Autodesk Inventor part; units mm, degrees
ref_plane "YZ Plane" through (0, 0, 0) normal (1, 0, 0) x (0, 1, 0)
ref_plane "XZ Plane" through (0, 0, 0) normal (0, 1, 0) x (-1, 0, 0)
ref_plane "XY Plane" through (0, 0, 0) normal (0, 0, 1) x (1, 0, 0)
sketch "スケッチ1" plane through (0, 0, 0) normal (0, 0, 1) x (1, 0, 0)
  line L0 (0, 0) -> (0, -3)
  line L1 (0, 0) -> (-15, 0)
  line L2 (-15, 0) -> (-15, -3)
  line L3 (-15, -3) -> (-30, -3)
  line L4 (-30, -3) -> (-30, 0)
  line L5 (-30, 0) -> (-45, 0)
  line L6 (-45, 0) -> (-45, -3)
  line L7 (-245.5996, 0) -> (-66.4062, 0)
  line L8 (-66.4062, 0) -> (-51.9242, -3.906)
  line L9 (-245.5996, 0) -> (-245.5996, -3)
  line L10 (-245.5996, -3) -> (-68.9626, -6)
  line L11 (-68.9626, -6) -> (-58.5737, -15.799)
  circle A0 centre (-53.7535, -10.6886) radius 4.025
  circle A1 centre (-53.7535, -10.6886) radius 1.5
  line L12 (0, -3) -> (0, -9)
  arc A2 (-54.2694, -3.6826) -> (-51.0532, -17.1739) centre (-53.7535, -10.6886) ccw
  line L13 (-54.2694, -3.6826) -> (-45, -3)
  line L14 (-51.0532, -17.1739) -> (-31.4218, -9)
  line L15 (-31.4218, -9) -> (0, -9)
  arc A3 (-46.7293, -10.7926) -> (-42.5418, -13.63) centre (-43.7046, -10.8374) ccw
  circle A4 centre (-43.7046, -10.8374) radius 1.5
  line L16 (-54.6828, -17.6519) -> (-41.7856, -19.3732)
  arc A5 (-41.7856, -19.3732) -> (-42.5418, -13.63) centre (-41.3887, -16.3996) ccw
  arc A6 (-58.5737, -15.799) -> (-54.6828, -17.6519) centre (-53.7535, -10.6886) ccw
  arc A7 (-46.7293, -10.7926) -> (-51.9242, -3.906) centre (-53.7535, -10.6886) ccw
  line L17 (-42, -3) -> (-33, -3)
  line L18 (-33, -3) -> (-33, -6)
  line L19 (-33, -6) -> (-42, -6)
  line L20 (-42, -6) -> (-42, -3)
  line L21 (-12, -3) -> (-3, -3)
  line L22 (-3, -3) -> (-3, -6)
  line L23 (-3, -6) -> (-12, -6)
  line L24 (-12, -6) -> (-12, -3)
  circle A8 centre (-40.95, -3) radius 1.05
  circle A9 centre (-34.05, -3) radius 1.05
  circle A10 centre (-34.05, -6) radius 1.05
  circle A11 centre (-40.95, -6) radius 1.05
  circle A12 centre (-10.95, -3) radius 1.05
  circle A13 centre (-4.05, -3) radius 1.05
  circle A14 centre (-4.05, -6) radius 1.05
  circle A15 centre (-10.95, -6) radius 1.05
  circle A16 centre (-28.95, -3) radius 1.05
  circle A17 centre (-16.05, -3) radius 1.05
  circle A18 centre (-41.3887, -16.3996) radius 1.25
  line L25 (-15.5802, -9) -> (-15.5802, -14)
  line L26 (-15.5802, -14) -> (-4.3492, -14)
  line L27 (-4.3492, -14) -> (-4.3492, -12)
  line L28 (-4.3492, -12) -> (-11.5802, -12)
  arc A19 (-11.5802, -9) -> (-11.5802, -12) centre (-11.5802, -10.5) ccw
  line L29 (-43.7046, -10.8374) -> (-53.7535, -10.6886)
  line L30 (-53.7535, -10.6886) -> (-43.8314, -9.0902)
  arc A20 (-43.0841, -6.159) -> (-46.8179, -9.5713) centre (-43.8314, -9.0902) ccw
  line L31 (-52.0181, -3.8813) -> (-43.0841, -6.159)
  circle A21 centre (-88, 0) radius 0.5
  circle A22 centre (-158, 0) radius 0.5
  circle A23 centre (-228, 0) radius 0.5
  point P0 (-5.1, -6)
  point P1 (-9.9, -6)
  point P2 (-12, -6)
  point P3 (-9.9, -3)
  point P4 (-5.1, -3)
  point P5 (-33, -3)
  point P6 (-33, -6)
  point P7 (-35.1, -6)
  point P8 (-39.9, -6)
  point P9 (-42, -6)
  point P10 (-42, -3)
  point P11 (-39.9, -3)
  point P12 (-35.1, -3)
  point P13 (-17.1, -3)
  point P14 (-27.9, -3)
  point P15 (-58.5737, -15.799)
  point P16 (-54.6828, -17.6519)
  point P17 (-51.9709, -3.8934)
  point P18 (-46.8179, -9.5713)
  point P19 (-87.5, 0)
  point P20 (-88.5, 0)
  point P21 (-157.5, 0)
  point P22 (-158.5, 0)
  point P23 (-227.5, 0)
  point P24 (-228.5, 0)
  dimension "d0" = 3
  dimension "d1" = 15
  dimension "d2" = 3
  dimension "d3" = 15
  dimension "d4" = 15
  dimension "d5" = 3
  dimension "d6" = 3
  dimension "d7" = 8.05
  dimension "d8" = 3
  dimension "d9" = 6
  dimension "d10" = 6
  dimension "d11" = 6.05
  dimension "d12" = 3
  dimension "d13" = 9
  dimension "d14" = 3
  dimension "d15" = 9
  dimension "d16" = 3
  dimension "d17" = 3
  dimension "d18" = 3
  dimension "d19" = 3
  dimension "d20" = 3
  dimension "d21" = 3
  dimension "d22" = 2.1
  dimension "d23" = 2.1
  dimension "d24" = 2.1
  dimension "d25" = 2.1
  dimension "d26" = 2.1
  dimension "d27" = 2.1
  dimension "d28" = 2.1
  dimension "d29" = 2.1
  dimension "d30" = 2.1
  dimension "d31" = 2.1
  dimension "d32" = 2.5
  dimension "d33" = 3
  dimension "d34" = 3
  dimension "d35" = 2
  dimension "d36" = 4
  dimension "d39" = 10
  dimension "d42" = 1
  dimension "d43" = 43
  dimension "d44" = 1
  dimension "d45" = 1
  dimension "d46" = 70
  dimension "d47" = 70
extrude "押し出し1" add sketch "スケッチ1" along normal blind 6 contours A5 L16 A2 L14 | L14 A2 L13 L8 A7 L30 A0 L29 A3 | L29 A0 L30 A7 | A7 L31 A20 | L11 L10 L9 L7 A23 A22 A21 L8 L13 A2
fillet "フィレット1" radius 1 1 edges at (-43.0841, -6.159, 3)
properties part number "シールド先端棒"
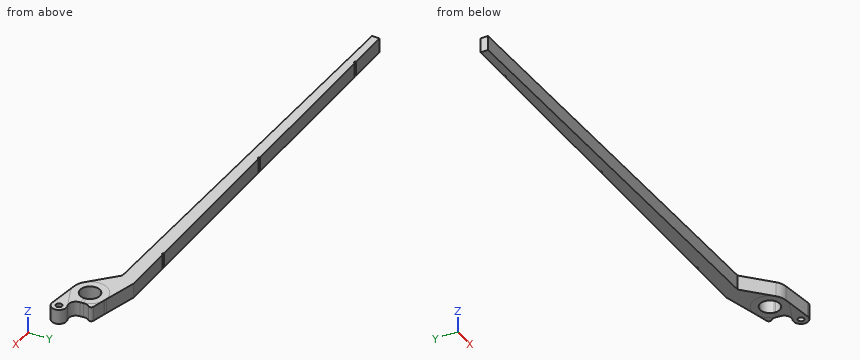
For this review, take the finished solid that the model builds, in its own axes (mm). Round coordinates to 2 decimals unless told otherwise and drop trailing zeros. Order: outer loops, then holes, each group sorted by start corner. A loop starts at its lowest first (then second) coordinate and runs counter-clockwise, first axis right, second up.
Q1. Wall thickness on line 1 (X direction, y = -9.75, z = 2.6); line 2 (X direction, y = -7, z = 1.65); line 3 (Y direction, x = -209.5, z = 5.45): over which ranges is each line inside the solid? List them lowest first.
Findings below:
line 1: x = -64.99 to -57.67, -49.84 to -46.79
line 2: x = -67.9 to -55.36, -52.14 to -46.02
line 3: y = -3.61 to 0
Q2. Insertion check: P1, Ø2, axis at x = -89, z = 5, coming from the -Y side; P2, Ø4, axis at x = -142.5, y = -5.5, coming from the -Z side. Each pin has a flat end and moves straight along its axis. Give the tip position at first contact, or say it passes through.
Findings below:
P1: stops at y = -5.68
P2: stops at z = 0
Q3. We need section A-A, the plane z = 3.6. State how many separate pieces and enclosed holes the cut face has, plus the area to 3 significant figures.
Findings below:
separate pieces: 1
enclosed holes: 2
area: 1,060 mm2
Q4. We need section C-C, the plane x = -84. Give the boundary of the cut face in (y, z), plus the area to 3 significant figures.
Findings below:
outline: (-5.74, 0) - (0, 0) - (0, 6) - (-5.74, 6) - close
area: 34.5 mm2
Q5. We need section B-B, the plane x = -220. Give the boundary of the cut face in (y, z), plus the area to 3 significant figures.
Findings below:
outline: (-3.43, 0) - (0, 0) - (0, 6) - (-3.43, 6) - close
area: 20.6 mm2
